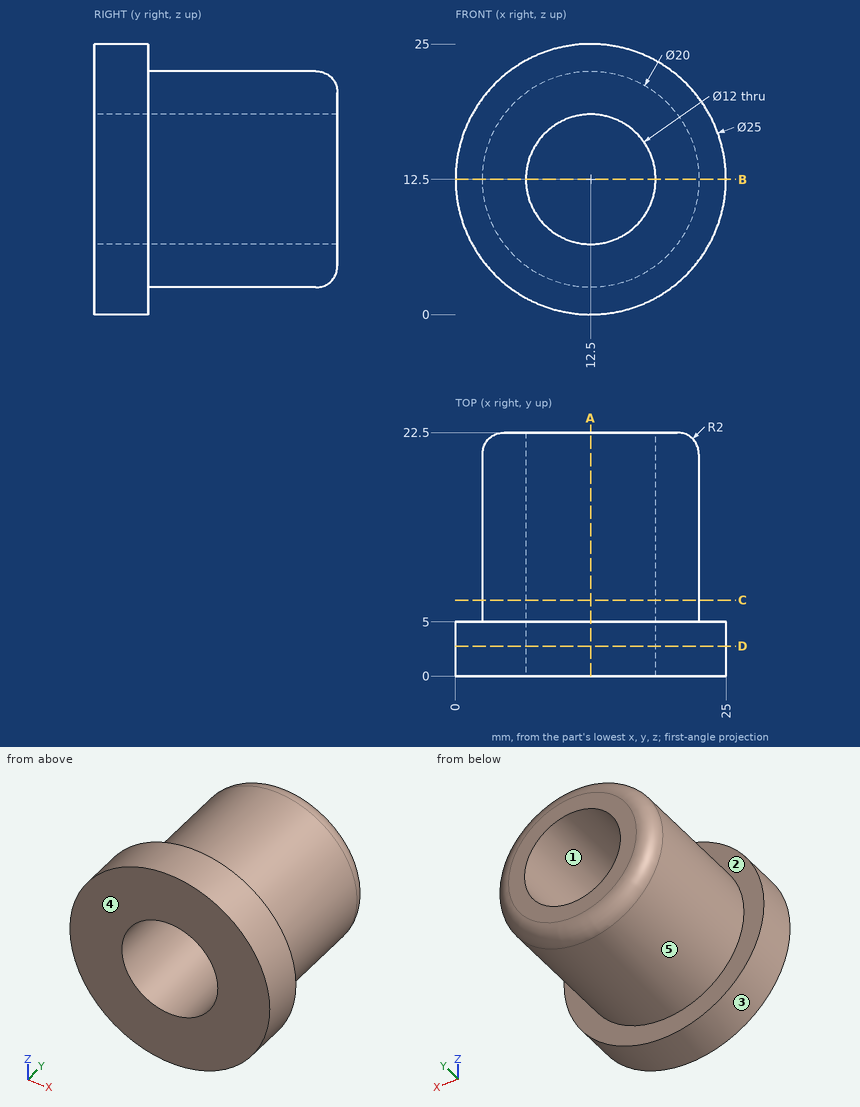
Answer from the drawing. Dimensions are ordinates in mm from the lowest x, y and z of the part. A direction names the side the tool comes from. Round coordinates to 2 decimals unless told otherwise and drop trailing zeros. Loops run counter-clockwise (first coordinate to the right, second up) from the corner with the lowest first, then second, coordinate; pieces in that order, holes last.
Q1. Section A-A on x = 12.5 is taken. Write down the section's boundary in (y, z).
Q2. Determine the mould class of the marked faces 1, 2 and 3 for opening direction X: released by +X, released by -X, zero draft, split by the parting line, or undercut.
Q3. Which of the six approach directions +Z, -Z, +X, -X, +Y, -Y give full straight-line access (tool end or side, diameter ignored) to the marked faces 4 and 5?
Q4. Section D-D on y = 2.75 is taken. Write down the section's boundary in (x, z), and give its area (3 significant figures).
Q5. Each of these flat-tipped pins is pushed along its axis until it touches: pin 1 (1 mm diameter, centred on y = 18.5, z = 5, fed in from -X); pin 2 (1.5 mm diameter, centred on x = 20.5, y = 16.5, fed in from +Z); pin 3 (1 mm diameter, centred on x = 14, y = 7, fed in from +Z); pin 4 (2 mm diameter, centred on x = 14, z = 20.5, fed in from +Y). Where does it stop, or does it pass through?
Q6. Consider probe 1 along Z at (x, y) = (12.5, 15.75); probe 2 along Y at (x, z) = (7.75, 22); probe 3 along Z at (x, y) = (14.75, 2.25). Determine where each line is inside the solid, lowest interval first.
Q7. Section C-C on y = 7 is taken. Write down the section's boundary in (x, z).
Q8. Section B-B on z = 12.5 is taken. Write down the section's boundary in (x, y), and give its area (3 significant figures).
Output:
1. outline: (0, 0) - (5, 0) - (5, 2.5) - (20.5, 2.5) arc R2 ccw to (22.5, 4.5) - (22.5, 6.5) - (0, 6.5) - close; (0, 18.5) - (22.5, 18.5) - (22.5, 20.5) arc R2 ccw to (20.5, 22.5) - (5, 22.5) - (5, 25) - (0, 25) - close
2. face 1: undercut
2. face 2: zero draft
2. face 3: split by the parting line
3. face 4: +Z, -Z, +X, -X, -Y
3. face 5: +Y
4. outline: circle Ø25 at (12.5, 12.5); hole circle Ø12 at (12.5, 12.5)
4. area: 378 mm2
5. pin 1: stops at x = 5.36
5. pin 2: stops at z = 19.39
5. pin 3: stops at z = 22.45
5. pin 4: stops at y = 22.5
6. probe 1: z = 2.5 to 6.5, 18.5 to 22.5
6. probe 2: y = 0 to 5
6. probe 3: z = 0.2 to 6.94, 18.06 to 24.8
7. outline: circle Ø20 at (12.5, 12.5); hole circle Ø12 at (12.5, 12.5)
8. outline: (0, 0) - (6.5, 0) - (6.5, 22.5) - (4.5, 22.5) arc R2 ccw to (2.5, 20.5) - (2.5, 5) - (0, 5) - close; (18.5, 0) - (25, 0) - (25, 5) - (22.5, 5) - (22.5, 20.5) arc R2 ccw to (20.5, 22.5) - (18.5, 22.5) - close
8. area: 203 mm2
